Can you work these out from the drawing? Everything is in mm from the part's minimum corner. A direction names the side the tool comes from. Round coordinates to 2 decimals unless told otherwise and drop trailing zeros. Loops run counter-clockwise (first coordinate to the right, second up) from the corner with the lowest first, then second, coordinate; pieces in that order, holes last. Notation, with made-up numbers: M 72.25,-24 L 124.25,-24 A22 cw 124.25,0 Z; hole C 35.5,56.5 d3. An arc over 180 degrees is marked long. Use a Markdown table: item, result.
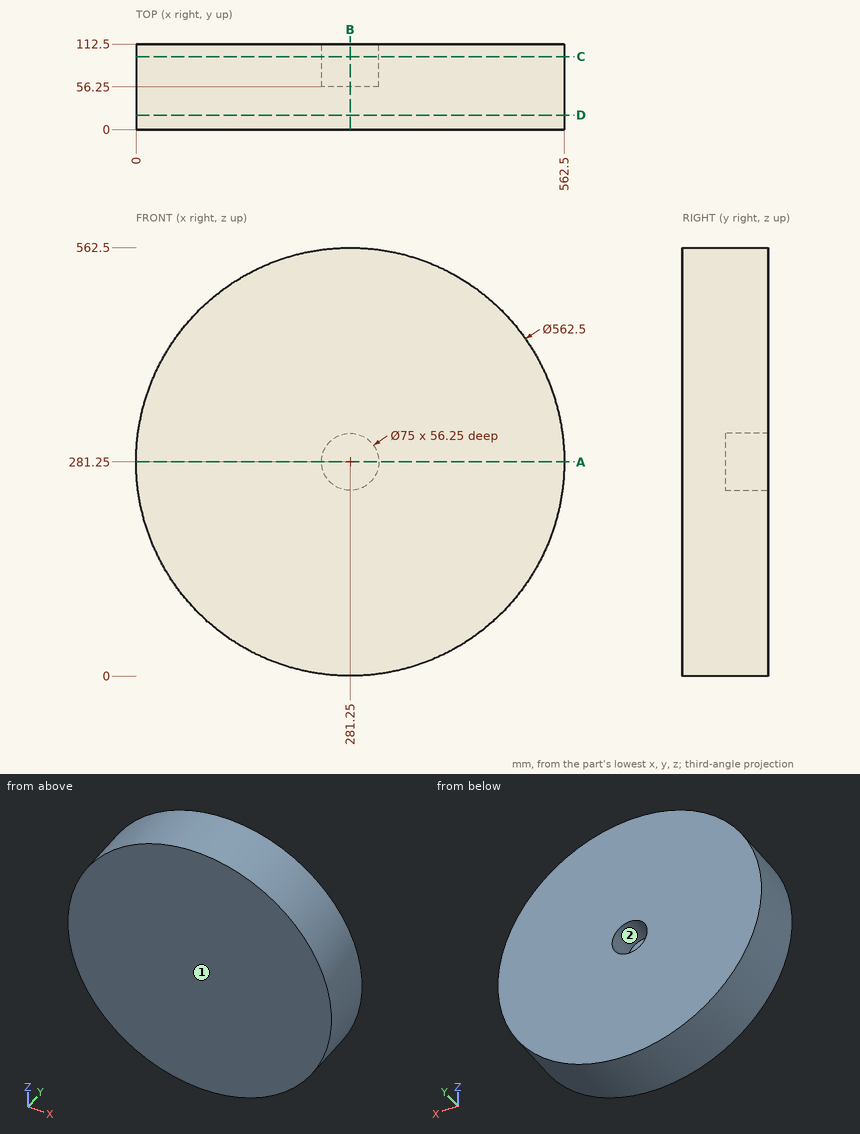
1. Imagine slicing it at A-A, the plane z = 281.25. Write out the boundary of the cut face in (x, y).
Answer sheet:
| item | result |
|---|---|
| outline | M 0,0 L 562.5,0 L 562.5,112.5 L 318.75,112.5 L 318.75,56.25 L 243.75,56.25 L 243.75,112.5 L 0,112.5 Z |
2. I need wall thicknesses on probe 1 along X at (y, z) = (101, 281.25); probe 2 along Z at (x, y) = (293, 93.5). Which ranges of each line are inside material? Lowest first, please. Write a range as from..to.
Answer sheet:
| item | result |
|---|---|
| probe 1 | 0..243.75, 318.75..562.5 |
| probe 2 | 0.25..245.64, 316.86..562.25 |
3. Imagine slicing it at D-D, the plane y = 19. Write out the boundary of the cut face in (x, z), then the cut area to 3 significant figures.
Answer sheet:
| item | result |
|---|---|
| outline | C 281.25,281.25 d562.5 |
| area | 249,000 mm2 |
4. For pin 1 Ø3 at (x, y) = (445.5, 100.5) entering from +Z; pin 2 Ø1.5 at (y, z) = (58.5, 303) entering from +X; pin 3 Ø2 at (y, z) = (49.5, 163) entering from +X, each with a flat end and sliding along its axis, tell me the tip position at first contact or that it passes through.
Answer sheet:
| item | result |
|---|---|
| pin 1 | z = 510.63 |
| pin 2 | x = 561.71 |
| pin 3 | x = 536.89 |
5. Imagine slicing it at B-B, the plane x = 281.25. Write out the boundary of the cut face in (y, z), then the cut area to 3 significant figures.
Answer sheet:
| item | result |
|---|---|
| outline | M 0,0 L 112.5,0 L 112.5,243.75 L 56.25,243.75 L 56.25,318.75 L 112.5,318.75 L 112.5,562.5 L 0,562.5 Z |
| area | 59,100 mm2 |
6. Which directions (+Z, -Z, +X, -X, +Y, -Y) give clear straight access to the entire face, cutting with the end or side of a thin tool? Please do the marked faces 1 and 2.
Answer sheet:
| item | result |
|---|---|
| face 1 | +Z, -Z, +X, -X, -Y |
| face 2 | +Y |
7. Imagine slicing it at C-C, the plane y = 96. Write out the boundary of the cut face in (x, z).
Answer sheet:
| item | result |
|---|---|
| outline | C 281.25,281.25 d562.5; hole C 281.25,281.25 d75 |
